Here's how the part is built. I have some questions about the finished solid (model axes, mm). Face numbers are marked on the shaded views. A direction names the side the tool comes from. Round coordinates to 2 decimals unless told otherwise and drop trailing zeros. Write each loop counter-clockwise with the first axis right and the second up, starting at its lowest first coordinate (ties: lowest second). Pieces come first, ordered by that corner, then holes. Notation, with made-up numbers: (8, -4.75) -> (54, -4.75) arc R28 cw to (54, 14.25) -> close; hole circle Ø5 at (44, 44.25). An arc over 180 degrees is marked (long way). Put each result on its own line as item: value. Start each with the question number.
1. Suppose I cut it at A-A (z = 0). Please give me the cut outline in (x, y), then the cut area to 3 significant figures.
2. Which directions (+Z, -Z, +X, -X, +Y, -Y) give clear straight access to the entire face, cutting with the end or side of a thin tool? Please do the marked faces 1, 2, 3 and 4.
3. Suppose I cut it at D-D (z = 3.5). Please give me the cut outline in (x, y), then the cut area to 3 significant figures.
4. We'd pull the mould along X, two halves only. Please class the marked faces 5, 6 and 7: +X half, -X half, draft (parallel to the pull), parting line (faces both ways), or undercut.
5. Suppose I cut it at C-C (x = -0.5). Please give me the cut outline in (y, z).
6. For pin 1 (1.5 mm diameter, centred on x = 4, y = 6, fed in from -Z); pin 2 (8 mm diameter, centred on y = 6.5, z = -4, fed in from +X); pin 3 (1.5 mm diameter, centred on x = 6.5, z = -0.5, fed in from -Y); pin 4 (4 mm diameter, centred on x = 5, z = 3, fed in from -Y), each with a flat end and sliding along its axis, tell me the tip position at first contact or that it passes through.
7. I need wall thicknesses on probe 1 along Y at (x, z) = (6, 3.5); probe 2 along Y at (x, z) = (18, 0); probe 3 along X at (y, z) = (-0.25, 1.25). Which ranges of each line are inside material? Lowest first, please. Write a range as from..to.
8. Suppose I cut it at B-B (x = 21.24). Please give me the cut outline in (y, z).
```python
from build123d import *

# Parameters (mm, degrees)
BOSS_EXTRUDE1_DEPTH = 5
CUT_EXTRUDE1_DEPTH  = 5
SKETCH3_R           = 5
BOSS_EXTRUDE2_DEPTH = 8
SKETCH5_R           = 4
BOSS_EXTRUDE4_DEPTH = 4


with BuildPart() as part:
    # Sketch1 → Boss-Extrude1 (new body)
    with BuildSketch(Plane(origin=(0, 0, 0), x_dir=(1, 0, 0), z_dir=(0, 1, 0))):
        with BuildLine():
            Line((0, 7), (22, 7))
            ThreePointArc((22, 7), (29, 0), (22, -7))
            Line((22, -7), (0, -7))
            ThreePointArc((0, -7), (-7, 0), (0, 7))
        make_face()
    extrude(amount=BOSS_EXTRUDE1_DEPTH)

    # Sketch2 → Cut-Extrude1 (cut)
    with BuildSketch(Plane(origin=(0, 5, 0), x_dir=(1, 0, 0), z_dir=(0, 1, 0))):
        with BuildLine():
            Line((1.5, 2), (1.5, -2))
            ThreePointArc((1.5, -2), (0, -2.5), (-1.5, -2))
            Line((-1.5, -2), (-1.5, 2))
            ThreePointArc((-1.5, 2), (0, 2.5), (1.5, 2))
        make_face()
    extrude(amount=-CUT_EXTRUDE1_DEPTH, mode=Mode.SUBTRACT)

    # Sketch3 → Boss-Extrude2 (add)
    with BuildSketch(Plane(origin=(0, 5, 0), x_dir=(1, 0, 0), z_dir=(0, 1, 0))):
        with Locations(Location((21.24, 0, 0), (0, 0, 270))):
            Circle(SKETCH3_R)
    extrude(amount=BOSS_EXTRUDE2_DEPTH)

    # Sketch5 → Boss-Extrude4 (add)
    with BuildSketch(Plane.XZ):
        with Locations(Location((0, 0, 0), (0, 0, 90))):
            Circle(SKETCH5_R)
        with BuildLine():
            Line((-1.5, 2), (-1.5, -2))
            ThreePointArc((-1.5, -2), (0, -2.5), (1.5, -2))
            Line((1.5, -2), (1.5, 2))
            ThreePointArc((1.5, 2), (0, 2.5), (-1.5, 2))
        make_face(mode=Mode.SUBTRACT)
    extrude(amount=BOSS_EXTRUDE4_DEPTH)


solid = part.part
```
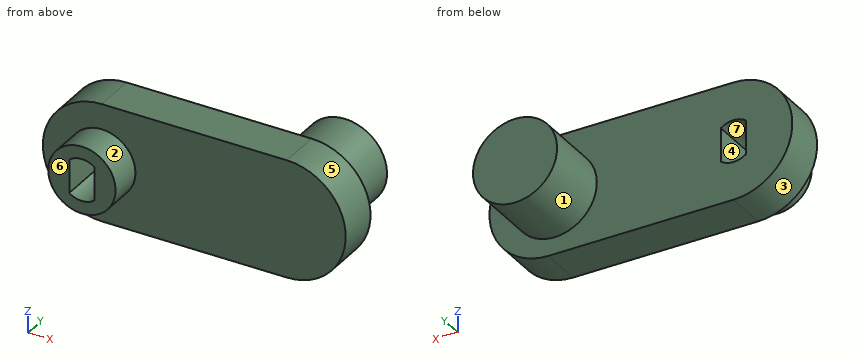
Verdict:
1. outline: (-7, 0) -> (-4, 0) -> (-4, -4) -> (-1.5, -4) -> (-1.5, 5) -> (-7, 5) -> close; (1.5, -4) -> (4, -4) -> (4, 0) -> (29, 0) -> (29, 5) -> (26.24, 5) -> (26.24, 13) -> (16.24, 13) -> (16.24, 5) -> (1.5, 5) -> close
1. area: 265 mm^2
2. face 1: +Y
2. face 2: -Y
2. face 3: -X, +Y, -Y
2. face 4: +Y, -Y
3. outline: (-6.06, 0) -> (-1.94, 0) -> (-1.94, -4) -> (1.94, -4) -> (1.94, 0) -> (28.06, 0) -> (28.06, 5) -> (24.81, 5) -> (24.81, 13) -> (17.67, 13) -> (17.67, 5) -> (-6.06, 5) -> close
3. area: 243 mm^2
4. face 5: +X half
4. face 6: draft
4. face 7: undercut
5. outline: (-4, -3.97) -> (0, -3.97) -> (0, -6.98) -> (5, -6.98) -> (5, -2.45) -> (-4, -2.45) -> close; (-4, 2.45) -> (5, 2.45) -> (5, 6.98) -> (0, 6.98) -> (0, 3.97) -> (-4, 3.97) -> close
6. pin 1: passes through
6. pin 2: stops at x = 28.99
6. pin 3: stops at y = 0
6. pin 4: stops at y = -4
7. probe 1: y = 0..5
7. probe 2: y = 0..13
7. probe 3: x = -3.8..-1.5, 1.5..3.8
8. outline: (0, -7) -> (5, -7) -> (5, -5) -> (13, -5) -> (13, 5) -> (5, 5) -> (5, 7) -> (0, 7) -> close
